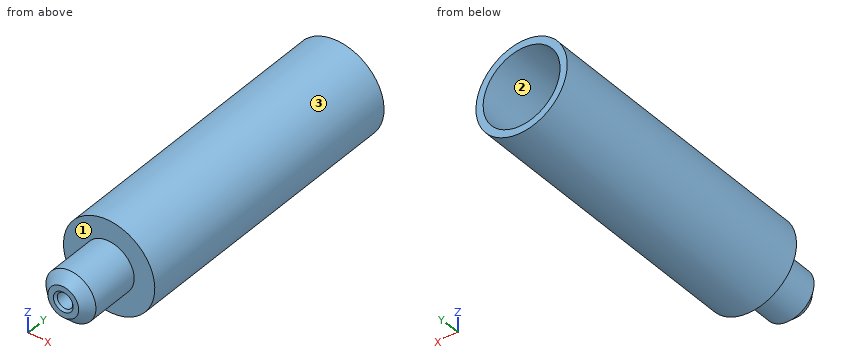
```python
from build123d import *

# Parameters (mm, degrees)
SKETCH1_R                   = 2.6
BOSS_EXTRUDE1_DEPTH         = 6
SKETCH2_R                   = 4.75
BOSS_EXTRUDE3_DEPTH         = 2.5
SKETCH3_R                   = 4.75
SKETCH3_R_2                 = 4
BOSS_EXTRUDE4_DEPTH         = 27.5
M2_TAPPED_HOLE1_D           = 1.6
M2_TAPPED_HOLE1_CSINK_D     = 2.05
M2_TAPPED_HOLE1_CSINK_ANGLE = 90
CHAMFER3_SIZE               = 1


with BuildPart() as part:
    # Sketch1 → Boss-Extrude1 (new body)
    with BuildSketch(Plane(origin=(0, 0, 0), x_dir=(1, 0, 0), z_dir=(0, 1, 0))):
        with Locations(Location((0, 0, 0), (0, 0, 270))):
            Circle(SKETCH1_R)
    extrude(amount=BOSS_EXTRUDE1_DEPTH)

    # Sketch2 → Boss-Extrude3 (add)
    with BuildSketch(Plane(origin=(0, 6, 0), x_dir=(1, 0, 0), z_dir=(0, 1, 0))):
        with Locations(Location((0, 0, 0), (0, 0, 270))):
            Circle(SKETCH2_R)
    extrude(amount=BOSS_EXTRUDE3_DEPTH)

    # Sketch3 → Boss-Extrude4 (add)
    with BuildSketch(Plane(origin=(0, 8.5, 0), x_dir=(1, 0, 0), z_dir=(0, 1, 0))):
        with Locations(Location((0, 0, 0), (0, 0, 270))):
            Circle(SKETCH3_R)
        with Locations(Location((0, 0, 0), (0, 0, 270))):
            Circle(SKETCH3_R_2, mode=Mode.SUBTRACT)
    extrude(amount=BOSS_EXTRUDE4_DEPTH)

    # M2 Tapped Hole1 (through all)
    with Locations(Plane(origin=(0, 0, 0), x_dir=(-1, 0, 0), z_dir=(0, -1, 0))):
        with Locations((0, 0)):
            CounterSinkHole(M2_TAPPED_HOLE1_D / 2, M2_TAPPED_HOLE1_CSINK_D / 2, counter_sink_angle=M2_TAPPED_HOLE1_CSINK_ANGLE)

    # Chamfer3
    chamfer3_edges = [part.edges().sort_by_distance(p)[0] for p in [
        (0, 0, -2.6),
    ]]
    chamfer(chamfer3_edges, length=CHAMFER3_SIZE)


solid = part.part
```
Input: part model. Units: mm. Frame: model coordinates. Face numbers are marked on the shaded views. Coordinates: 2 decimals unless noted, no trailing zeros. Write each loop counter-clockwise with the first axis right and the second up, starting at its lowest first coordinate (ties: lowest second). Pieces come first, ordered by that corner, then holes. Notation, with made-up numbers: (14, 10) - (68, 10) arc R24 ccw to (68, 34) - close; hole circle Ø8 at (-13.5, 72.25). An arc over 180 degrees is marked (long way). Put each result on its own line as item: value. Start each with the question number.
1) Cut plane C-C (y = 30). Return the cut outline in (x, z).
2) Ray query, L1, parallel to X at y = 26, z = 0; L2, parallel to Y at x = 1, z = 3; L3, parallel to Z at x = 3.5, y = 15. Return the intervals inside material, ascending.
3) Cut plane B-B (z = 0). Return the cut outline in (x, y) (3 decimals).
4) Mould query, pull axis X, two halves, no side actions, for the marked faces 1, 2 and 3. Classes: pulls with the +X half, pulls with the -X half, needs draft (parallel to the pull), parting line crosses it, or undercut.
5) Cut plane D-D (x = 3.5). Return the cut outline in (y, z).
6) Contact query for flat-ended pins moving along their axis: pin 1 (4 mm diameter, centred on x = -1, z = -0.5, fed in from +Y); pin 2 (1.5 mm diameter, centred on y = 4.5, z = 1, fed in from +X); pin 3 (1 mm diameter, centred on x = 0, z = 0, fed in from +Y); pin 4 (1.5 mm diameter, centred on x = 3.5, y = 19.5, fed in from +Z). Output: stop coordinate, or through.
7) Cut plane A-A (x = 0). Return the cut outline in (y, z) (3 decimals).
Resolved:
1. outline: circle Ø9.5 at (0, 0); hole circle Ø8 at (0, 0)
2. L1: x = -4.75 to -4, 4 to 4.75
2. L2: y = 6 to 8.5
2. L3: z = -3.21 to -1.94, 1.94 to 3.21
3. outline: (-4.75, 6) - (-2.6, 6) - (-2.6, 1) - (-1.6, 0) - (-1.025, 0) - (-0.8, 0.225) - (-0.8, 8.5) - (-4, 8.5) - (-4, 36) - (-4.75, 36) - close; (0.8, 0.225) - (1.025, 0) - (1.6, 0) - (2.6, 1) - (2.6, 6) - (4.75, 6) - (4.75, 36) - (4, 36) - (4, 8.5) - (0.8, 8.5) - close
4. face 1: needs draft
4. face 2: undercut
4. face 3: parting line crosses it
5. outline: (6, -3.21) - (36, -3.21) - (36, -1.94) - (8.5, -1.94) - (8.5, 1.94) - (36, 1.94) - (36, 3.21) - (6, 3.21) - close
6. pin 1: stops at y = 8.5
6. pin 2: stops at x = 2.59
6. pin 3: passes through
6. pin 4: stops at z = 3.87
7. outline: (0, -1.6) - (1, -2.6) - (6, -2.6) - (6, -4.75) - (36, -4.75) - (36, -4) - (8.5, -4) - (8.5, -0.8) - (0.225, -0.8) - (0, -1.025) - close; (0, 1.025) - (0.225, 0.8) - (8.5, 0.8) - (8.5, 4) - (36, 4) - (36, 4.75) - (6, 4.75) - (6, 2.6) - (1, 2.6) - (0, 1.6) - close
